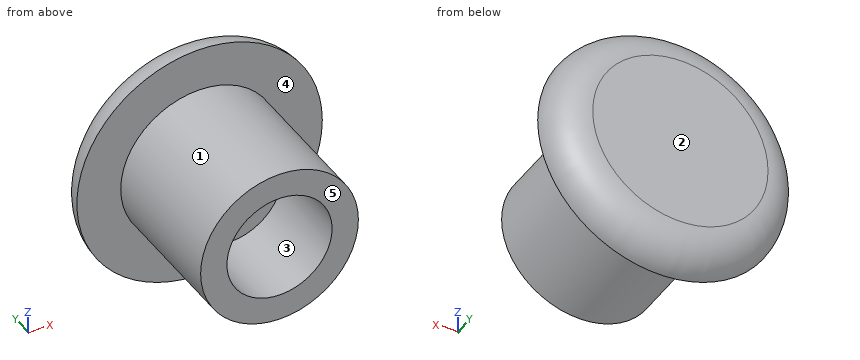
```python
from build123d import *

# Parameters (mm, degrees)
F0_R     = 4.5
F1_DEPTH = 8
F0_R_2   = 7
F2_DEPTH = 2
F3_R     = 1.99999
F4_R     = 3
F5_DEPTH = 5


# Not quite as in the source:
# - a fillet or chamfer is up to 0.001 mm smaller than in the source, because OpenCascade refuses the exact size


with BuildPart() as f1:
    # F0 (on Front) → F1 (new body)
    with BuildSketch(Plane.XZ):
        Circle(F0_R)
    extrude(amount=F1_DEPTH)

    # F0 (on Front) → F2 (join)
    with BuildSketch(Plane.XZ):
        Circle(F0_R_2)
        Circle(F0_R, mode=Mode.SUBTRACT)
        Circle(F0_R)
    extrude(amount=-F2_DEPTH)

    # F3 (radius 2 in the source; OpenCascade refuses exactly that, so slightly less here)
    f3_edges = [f1.edges().sort_by_distance(p)[0] for p in [
        (-7, 2, 0),
    ]]
    fillet(f3_edges, radius=F3_R)

    # F4 (on face) → F5 (cut)
    with BuildSketch(Plane.XZ.offset(8)):
        Circle(F4_R)
    extrude(amount=-F5_DEPTH, mode=Mode.SUBTRACT)


solid = f1.part
```
Check sheet for the modelled part. Datum: model origin and axes. Units: mm. Face numbers are marked on the shaded views. A direction names the side the tool comes from. Give positions to 0.01 mm unless a question says otherwise; leave off trailing zeros. Order: outer loops, then holes, each group sorted by start corner. A loop starts at its lowest first (then second) coordinate and runs counter-clockwise, first axis right, second up. Notation, with made-up numbers: M 26.5,-11 L 44.5,-11 A19 cw 44.5,0 Z; hole C 73,88 d1. An arc over 180 degrees is marked long. Answer in a Markdown table with one row per item.
1) Cross-section at D-D, the plane y = 0.75. Enter the section's corners in (x, z), plus the area to 3 significant figures.
Filled sheet:
| item | result |
|---|---|
| outline | C 0,0 d13.71 |
| area | 148 mm2 |
2) Thickness scan on L1, parallel to Z at x = 0, y = -5.95; L2, parallel to Y at x = 4.5, z = 1.75; L3, parallel to Y at x = 2.75, z = -0.5. Record the ranges inside material, lowest first. Write a range as [from, to].
Filled sheet:
| item | result |
|---|---|
| L1 | z = [-4.5, -3], [3, 4.5] |
| L2 | y = [0, 2] |
| L3 | y = [-3, 2] |
3) Release check for a two-part mould opening along X. For the marked faces 1, 2 and 3 record: +X half, -X half, draft (parallel to the pull), parting line (faces both ways), or undercut.
Filled sheet:
| item | result |
|---|---|
| face 1 | parting line |
| face 2 | draft |
| face 3 | undercut |
4) Cross-section at C-C, the plane y = -4.25. Enter the section's corners in (x, z).
Filled sheet:
| item | result |
|---|---|
| outline | C 0,0 d9; hole C 0,0 d6 |
5) Access from +Z, -Z, +X, -X, +Y, -Y to the whole of each face (thin tool, end or side, straight path). Record for the marked faces 4 and 5.
Filled sheet:
| item | result |
|---|---|
| face 4 | -Y |
| face 5 | +Z, -Z, +X, -X, -Y |
6) Gauge pin test, flat ends, axial feed: P1, Ø1, axis at x = -2, z = 5.5, coming from the +Y side; P2, Ø1.5, axis at x = 1.5, y = -2, coming from the +Z side; P3, Ø7, axis at x = 0, z = 0, coming from the -Y side; P4, Ø1, axis at y = -3, z = -5.5, coming from the -X side. Record the tip position at first contact, or that the pin passes through.
Filled sheet:
| item | result |
|---|---|
| P1 | stops at y = 1.97 |
| P2 | stops at z = 4.44 |
| P3 | stops at y = -8 |
| P4 | passes through |
